```python
from build123d import *

# Parameters (mm, degrees)
F1_DEPTH = 15
F2_R     = 3
F3_R     = 2.5
F4_DEPTH = 2.001
F5_R     = 5
F6_R     = 1
F7_R     = 2.6650989984
F8_DEPTH = 2.001


# Not quite as in the source:
# - a pattern or mirror of a feature is missing from the dataset's text; its kind, count and spacing are read off the source's solid


with BuildPart() as f1:
    # F0 (on Front) → F1 (new body, symmetric)
    with BuildSketch(Plane.XZ):
        Polygon((-30, 2), (-30, 0), (0, 0), (0, 30), (-2, 30), (-2, 2), align=None)
    extrude(amount=F1_DEPTH, both=True)

    # F2
    f2_edges = [f1.edges().sort_by_distance(p)[0] for p in [
        (0, 0, 0),
        (-2, 0, 2),
    ]]
    fillet(f2_edges, radius=F2_R)

    # F3 (on face) → F4 (cut, through all)
    with BuildSketch(Plane.XY.offset(2)):
        with Locations((-20, 7)):
            Circle(F3_R)
        with Locations((-20, -7)):
            Circle(F3_R)
    extrude(amount=-F4_DEPTH, mode=Mode.SUBTRACT)

    # F5
    f5_edges = [f1.edges().sort_by_distance(p)[0] for p in [
        (-30, -15, 1),
        (-30, 15, 1),
        (-1, -15, 30),
        (-1, 15, 30),
    ]]
    fillet(f5_edges, radius=F5_R)

    # F6
    f6_edges = [f1.edges().sort_by_distance(p)[0] for p in [
        (-15, 15, 2),
        (-28.535534, 13.535534, 2),
        (-30, 0, 2),
        (-15, -15, 2),
        (-28.535534, -13.535534, 2),
        (-2.87868, 15, 2.87868),
        (-2, 15, 15),
        (-2.87868, -15, 2.87868),
        (-2, -15, 15),
        (-2, 13.535534, 28.535534),
        (-2, 0, 30),
        (-2, -13.535534, 28.535534),
    ]]
    fillet(f6_edges, radius=F6_R)

    # F7 (on face) → F8 (cut, through all)
    with BuildSketch(Plane(origin=(-2, 0, 0), x_dir=(0, -1, 0), z_dir=(-1, 0, 0))):
        with Locations((-7, 20)):
            Circle(F7_R)
    f8 = extrude(amount=-F8_DEPTH, mode=Mode.SUBTRACT)

    # F8_copies: F8 across plane
    add(f8.mirror(Plane(origin=(0, 0, 0), x_dir=(0, 0, -1), z_dir=(0, -1, 0))), mode=Mode.SUBTRACT)


solid = f1.part
```
Source: CAD feature listing. Evaluate the final solid. Frame: model axes, mm. A direction names the side the tool comes from. Coordinates: 2 decimals unless noted, no trailing zeros. Write each loop counter-clockwise with the first axis right and the second up, starting at its lowest first coordinate (ties: lowest second). Pieces come first, ordered by that corner, then holes. Notation, with made-up numbers: (28, 44.5) - (71, 44.5) arc R24 cw to (71, 67.5) - close; hole circle Ø2 at (18, 16.25). An arc over 180 degrees is marked (long way). Answer as a JSON object with one key per item and string values.
Q1. Section query C-C, the plane x = -20. Output: boundary loops of the cut face in (y, z), plus the area to 3 significant figures.
Ans:
{"outline": "(-15, 0) - (-9.5, 0) - (-9.5, 2) - (-14, 2) arc R1 ccw to (-15, 1) - close; (-4.5, 0) - (4.5, 0) - (4.5, 2) - (-4.5, 2) - close; (9.5, 0) - (15, 0) - (15, 1) arc R1 ccw to (14, 2) - (9.5, 2) - close", "area": "39.6 mm2"}
Q2. Material intervals for line 1 (Y direction, x = -20, z = 1.15); line 2 (Y direction, x = -20, z = 1.35); line 3 (X direction, y = 5, z = 9), sorted ascending. Write a range as [from, to].
Ans:
{"line 1": "y = [-14.99, -9.5], [-4.5, 4.5], [9.5, 14.99]", "line 2": "y = [-14.94, -9.5], [-4.5, 4.5], [9.5, 14.94]", "line 3": "x = [-2, 0]"}
Q3. Section query A-A, the plane z = 20. Output: boundary loops of the cut face in (x, y).
Ans:
{"outline": "(-2, -14) arc R1 ccw to (-1, -15) - (0, -15) - (0, -9.67) - (-2, -9.67) - close; (-2, -4.33) - (0, -4.33) - (0, 4.33) - (-2, 4.33) - close; (-2, 9.67) - (0, 9.67) - (0, 15) - (-1, 15) arc R1 ccw to (-2, 14) - close"}
Q4. Section query D-D, the plane x = -13.75. Output: boundary loops of the cut face in (y, z), plus the area to 3 significant figures.
Ans:
{"outline": "(-15, 0) - (15, 0) - (15, 1) arc R1 ccw to (14, 2) - (-14, 2) arc R1 ccw to (-15, 1) - close", "area": "59.6 mm2"}
Q5. Section query B-B, the plane y = 7. Output: boundary loops of the cut face in (x, z), plus the area to 3 significant figures.
Ans:
{"outline": "(-30, 0) - (-22.5, 0) - (-22.5, 2) - (-29, 2) arc R1 ccw to (-30, 1) - close; (-17.5, 0) - (-3, 0) arc R3 ccw to (0, 3) - (0, 17.33) - (-2, 17.33) - (-2, 5) arc R3 cw to (-5, 2) - (-17.5, 2) - close; (-2, 22.67) - (0, 22.67) - (0, 30) - (-1, 30) arc R1 ccw to (-2, 29) - close", "area": "94.9 mm2"}
Q6. Set-up query: faces 4 (the flat face through (-30, -0.1, 0.5)), 5 (the cylindrical face through (-1.715, -14.699, 15.14)), 6 (the cylindrical face through (-1.715, 14.699, 14.86)). Return all of +Z, -Z, +X, -X, +Y, -Y with unobstructed straight access to the full face (end or side cutting, diameter ignored); none if empty.
Ans:
{"face 4": "+Z, -Z, -X, +Y, -Y", "face 5": "+Z, -X, -Y", "face 6": "+Z, -X, +Y"}
Q7. First-contact query: pin 1 Ø1.5 at (y, z) = (3, 15.5) entering from -X; pin 2 Ø5 at (x, y) = (-18.5, -6) entering from +Z. Flat tips, straight axial feed; report the tip coordinate or a pass-through.
Ans:
{"pin 1": "stops at x = -2", "pin 2": "stops at z = 2"}
Q8. Draft query along X for faces 1 (the flat face through (-2, 0, 17)), 2 (the cylindrical face through (-22.5, -6.9, 1)), 3 (the flat face through (-0.5, -15, 6.1)). Return one class per face: released by +X, released by -X, zero draft, split by the parting line, or undercut.
Ans:
{"face 1": "released by -X", "face 2": "undercut", "face 3": "zero draft"}
